Verification items for this drawing (mm, ordinates from the low corner). A direction names the side the tool comes from. Round coordinates to 2 decimals unless told otherwise and drop trailing zeros. Order: outer loops, then holes, each group sorted by start corner. A loop starts at its lowest first (then second) coordinate and runs counter-clockwise, first axis right, second up. Notation, with made-up numbers: (-1.75, -10.75) -> (48.25, -10.75) arc R27 cw to (48.25, 23.25) -> close; hole circle Ø1 at (41, -36.75). An arc over 180 degrees is marked (long way). Return JSON: item names as keys, results as strings. Group by question number.
Item 1: Sectioned sample at B-B on x = 31.5. Record the cut outline in (y, z).
Item 2: Depth check by flat-ended pin: pin 1 Ø10 at (y, z) = (22.5, 29) entering from -X (1 decimal); pin 2 Ø11 at (x, z) = (35, 30) entering from +Y; pin 3 Ø11 at (x, z) = (32.5, 34.5) entering from -Y; pin 4 Ø8 at (x, y) = (31.5, 32) entering from -Z. Enter the tip coordinate at first touch or a pass-through.
Item 3: Sectioned sample at C-C on z = 37.5. Record the cut outline in (x, y) (1 decimal).
Item 4: Scan lines: probe 1 along Y at (x, z) = (37, 26); probe 2 along Z at (x, y) = (46, 20); probe 3 along Y at (x, z) = (12.5, 16). Record each from-to range of solid material in increasing order. Write a range as from..to.
Item 5: Sectioned sample at A-A on y = 21.5. Record the cut outline in (x, z) (1 decimal), plus the area to 3 significant figures.
Item 6: Access from +Z, -Z, +X, -X, +Y, -Y to the whole of each face (thin tool, end or side, straight path). Record for the marked faces 1, 2 and 3.
Item 7: Sectioned sample at D-D on y = 36. Record the cut outline in (x, z), plus the area to 3 significant figures.
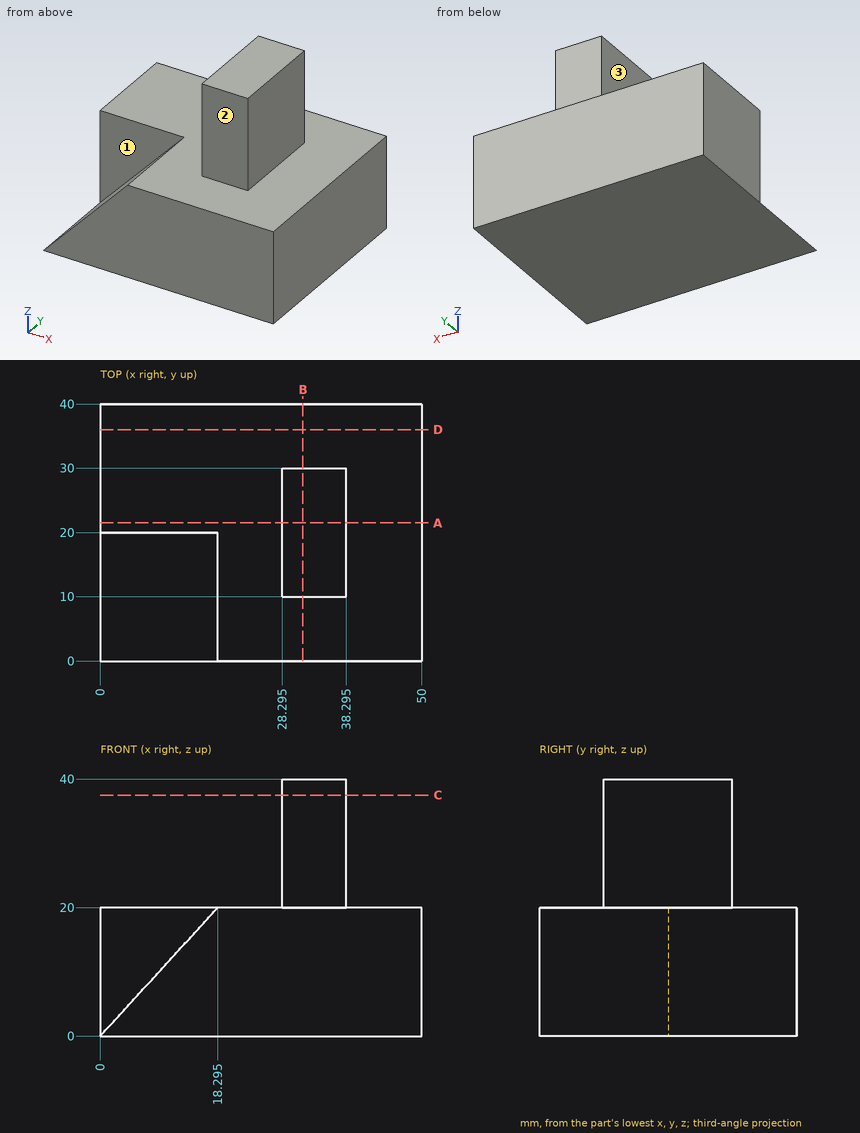
Recorded:
{
 "1": {"outline": "(0, 0) -> (40, 0) -> (40, 20) -> (30, 20) -> (30, 40) -> (10, 40) -> (10, 20) -> (0, 20) -> close"},
 "2": {"pin 1": "x = 28.3", "pin 2": "y = 30", "pin 3": "y = 10", "pin 4": "z = 0"},
 "3": {"outline": "(28.3, 10) -> (38.3, 10) -> (38.3, 30) -> (28.3, 30) -> close"},
 "4": {"probe 1": "10..30", "probe 2": "0..20", "probe 3": "20..40"},
 "5": {"outline": "(0, 0) -> (50, 0) -> (50, 20) -> (38.3, 20) -> (38.3, 40) -> (28.3, 40) -> (28.3, 20) -> (0, 20) -> close", "area": "1,200 mm²"},
 "6": {"face 1": "+Z, -X, -Y", "face 2": "+Z, +X, -X, -Y", "face 3": "+Z, -X, +Y, -Y"},
 "7": {"outline": "(0, 0) -> (50, 0) -> (50, 20) -> (0, 20) -> close", "area": "1,000 mm²"}
}
